Check sheet for the modelled part. Datum: model origin and axes. Units: mm. A direction names the side the tool comes from. Give positions to 0.01 mm unless a question says otherwise; leave off trailing zeros. Write each loop counter-clockwise with the first axis right and the second up, starting at its lowest first coordinate (ties: lowest second). Pieces come first, ordered by that corner, then holes. Notation, with made-up numbers: M -10,59 L 10,59 A15 cw 10,74 Z; hole C 4,-40 d11. An arc over 180 degrees is marked long. One line per item, written item: value. Start each with the question number.
Autodesk Inventor part; units mm, degrees
ref_plane "1_XY" through (0, 0, 0) normal (0, 1, 0) x (1, 0, 0)
ref_plane "1_YZ" through (0, 0, 0) normal (1, 0, 0) x (0, 0, -1)
ref_plane "1_ZX" through (0, 0, 0) normal (0, 0, -1) x (0, 1, 0)
sketch "Sketch_1" plane through (0, 0, 0) normal (0, 0, 1) x (1, 0, 0)
  line L0 (0, -39.9) -> (0, 36.8)
  line L1 (0, 36.8) -> (2, 36.8)
  line L2 (2, 36.8) -> (2.5, 36.3)
  line L3 (2.5, 36.3) -> (2.5, 0)
  line L4 (2.5, 0) -> (4.4, 0)
  line L5 (4.4, 0) -> (4.4, -0.85)
  line L6 (4.4, -0.85) -> (4.5, -0.85)
  line L7 (4.5, -0.85) -> (4.5, -1.7)
  line L8 (4.5, -1.7) -> (5.5, -1.7)
  line L9 (5.5, -1.7) -> (5.5, -36.7)
  line L10 (5.5, -36.7) -> (4.5, -36.7)
  line L11 (4.5, -36.7) -> (4.5, -37.55)
  line L12 (4.5, -37.55) -> (4.4, -37.55)
  line L13 (4.4, -37.55) -> (4.4, -38.4)
  line L14 (4.4, -38.4) -> (2.5, -38.4)
  line L15 (2.5, -38.4) -> (2.5, -39.4)
  line L16 (2.5, -39.4) -> (2, -39.9)
  line L17 (2, -39.9) -> (0, -39.9)
  line L18 (0, -39.9) -> (0, 36.8)
revolve "Revolution1" add sketch "Sketch_1" angle 360 about axis through (0, -39.9, 0) along (0, -1, 0)
sketch "Sketch_2" plane through (0, 0, 5.5) normal (0, 0, 1) x (1, 0, 0)
  line L0 (0, -36.7) -> (24, -36.7)
  line L1 (24, -36.7) -> (24, -1.7)
  line L2 (24, -1.7) -> (0, -1.7)
  line L3 (0, -1.7) -> (0, -36.7)
extrude "Extrusion1" add sketch "Sketch_2" against normal blind 3.5
sketch "Sketch3" plane through (0, 0, 5.5) normal (0, 0, 1) x (1, 0, 0)
  point P0 (16, -9.2)
hole "Hole1" at (16, -9.2, 5.5) direction (0, 0, -1) diameter 5.5 depth 3.5 countersink diameter 11 countersink angle 90
sketch "Sketch4" plane through (0, 0, 5.5) normal (0, 0, 1) x (1, 0, 0)
  point P0 (16, -29.2)
hole "Hole2" at (16, -29.2, 5.5) direction (0, 0, -1) diameter 5.5 depth 3.5 countersink diameter 11 countersink angle 90
ref_plane "1_XY" through (0, 0, 0) normal (0, 1, 0) x (1, 0, 0)
ref_plane "1_YZ" through (0, 0, 0) normal (1, 0, 0) x (0, 0, -1)
ref_plane "1_ZX" through (0, 0, 0) normal (0, 0, -1) x (0, 1, 0)
ref_plane "to_bolt1_XY" through (16, -9.2, 5.5) normal (0, 0, 1) x (1, 0, 0)
ref_plane "to_bolt1_YZ" through (16, -9.2, 5.5) normal (1, 0, 0) x (0, 1, 0)
ref_plane "to_bolt1_ZX" through (16, -9.2, 5.5) normal (0, 1, 0) x (0, 0, 1)
ref_plane "to_bolt1_r_XY" through (-16, -9.2, 5.5) normal (0, 0, 1) x (1, 0, 0)
ref_plane "to_bolt1_r_YZ" through (-16, -9.2, 5.5) normal (1, 0, 0) x (0, 1, 0)
ref_plane "to_bolt1_r_ZX" through (-16, -9.2, 5.5) normal (0, 1, 0) x (0, 0, 1)
ref_plane "to_bolt2_XY" through (16, -29.2, 5.5) normal (0, 0, 1) x (1, 0, 0)
ref_plane "to_bolt2_YZ" through (16, -29.2, 5.5) normal (1, 0, 0) x (0, 1, 0)
ref_plane "to_bolt2_ZX" through (16, -29.2, 5.5) normal (0, 1, 0) x (0, 0, 1)
ref_plane "to_bolt2_r_XY" through (-16, -29.2, 5.5) normal (0, 0, 1) x (1, 0, 0)
ref_plane "to_bolt2_r_YZ" through (-16, -29.2, 5.5) normal (1, 0, 0) x (0, 1, 0)
ref_plane "to_bolt2_r_ZX" through (-16, -29.2, 5.5) normal (0, 1, 0) x (0, 0, 1)
properties part number "HHPFLN5-1"
1) Tool access check on faces 1 (the cylindrical face through (14.141, -7.173, 2.37)), 2 (the cylindrical face through (-0.59, -37.13, 4.46)), 3 (the cylindrical face through (4.197, -0.431, 1.322)). Record the directions out of +Z, -Z, +X, -X, +Y, -Y that give a thin tool (end or side, any length) a straight path to the whole face; none if there is none.
2) Cross-section at B-B (x = 16). Record the boundary of the cut face in (y, z).
3) Cross-section at A-A (y = -29.2). Record the boundary of the cut face in (x, z), plus the area to 3 significant figures.
4) Gauge pin test, flat ends, axial feed: pin 1 (3.5 mm diameter, centred on x = 8, z = 1, fed in from +Y); pin 2 (5 mm diameter, centred on x = 3, y = 24, fed in from -Z); pin 3 (5.5 mm diameter, centred on x = 11.5, y = -27.5, fed in from -Z). Record the tip position at first contact, or that the pin passes through.
5) Cross-section at D-D (x = 9.25). Record the boundary of the cut face in (y, z), plus the area to 4 significant figures.
6) Material ranges on L1, parallel to Y at x = 16, z = 2.5; L2, parallel to Y at x = 11.5, z = 3.5; L3, parallel to X at y = -9.2, z = 2.5, recorded low to high. Write a range as from..to.
7) Draft check along Y on faces 4 (the flat face through (10.3, -1.7, 2.5)), 5 (the cylindrical face through (-0.54, -38.91, -2.44)), 6 (the cylindrical face through (15.17, -31.82, 2.37)), 7 (the conical face through (14.881, -31.899, 2.922)). Enter one of: released by +Y, released by -Y, zero draft, split by the parting line, or undercut.
Data:
1. face 1: +Z, -Z
1. face 2: -Y
1. face 3: +Y
2. outline: M -36.7,2 L -31.95,2 L -31.95,2.75 L -34.7,5.5 L -36.7,5.5 Z; M -26.45,2 L -11.95,2 L -11.95,2.75 L -14.7,5.5 L -23.7,5.5 L -26.45,2.75 Z; M -6.45,2 L -1.7,2 L -1.7,5.5 L -3.7,5.5 L -6.45,2.75 Z
3. outline: M 0,5.5 A5.5 ccw long 5.12,2 L 13.25,2 L 13.25,2.75 L 10.5,5.5 Z; M 18.75,2 L 24,2 L 24,5.5 L 21.5,5.5 L 18.75,2.75 Z
3. area: 139 mm2
4. pin 1: stops at y = -1.7
4. pin 2: stops at z = -2.45
4. pin 3: stops at z = 2
5. outline: M -36.7,2 L -1.7,2 L -1.7,5.5 L -36.7,5.5 Z
5. area: 122.5 mm2
6. L1: y = -36.7..-31.95, -26.45..-11.95, -6.45..-1.7
6. L2: y = -36.7..-1.7
6. L3: x = -4.9..13.25, 18.75..24
7. face 4: released by +Y
7. face 5: zero draft
7. face 6: undercut
7. face 7: undercut
